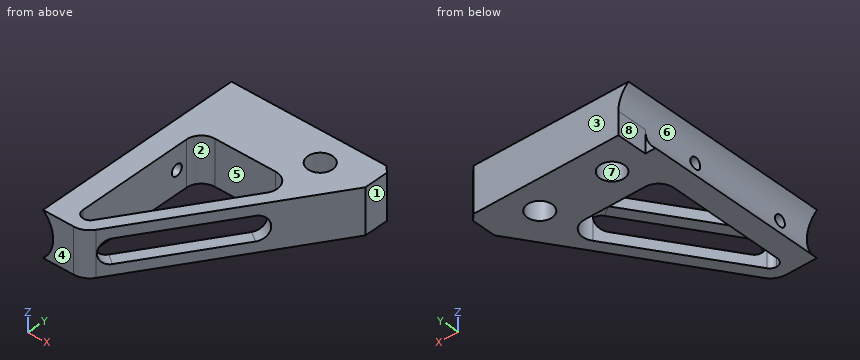
from build123d import *

# Parameters (mm, degrees)
P_IDAT_VYSUNUT_M1_DEPTH  = 15
SKICA3_R                 = 4.1
ODEBRAT_VYSUNUT_M1_DEPTH = 88.321245983
SKICA4_R                 = 4.05
ODEBRAT_VYSUNUT_M2_DEPTH = 10
ODEBRAT_VYSUNUT_M3_DEPTH = 88.321245983
P_IDAT_VYSUNUT_M2_DEPTH  = 70
SKICA7_W                 = 3.385621722
SKICA7_H                 = 7.5
ODEBRAT_VYSUNUT_M5_DEPTH = 10
SKICA9_W                 = 8
SKICA9_H                 = 44.544482181
ODEBRAT_VYSUNUT_M6_DEPTH = 88.290898193
ZAOBLIT2_R               = 4
SKICA10_R                = 1.85
ODEBRAT_VYSUNUT_M7_DEPTH = 86.094065598
ZAOBLIT7_R               = 6
ZKOSEN_1_SIZE            = 2


with BuildPart() as part:
    # Skica1 → Přidat vysunutím1 (new body)
    with BuildSketch(Plane.XY):
        Polygon((0, 0), (0, 70), (50, 70), (50, 60), (10, 0), align=None)
    extrude(amount=P_IDAT_VYSUNUT_M1_DEPTH)

    # Skica3 → Odebrat vysunutím1 (cut, through all)
    with BuildSketch(Plane.XY.offset(15)):
        with Locations((35, 60)):
            Circle(SKICA3_R)
    extrude(amount=-ODEBRAT_VYSUNUT_M1_DEPTH, mode=Mode.SUBTRACT)

    # Skica4 → Odebrat vysunutím2 (cut)
    with BuildSketch(Plane(origin=(0, 0, 0), x_dir=(-1, 0, 0), z_dir=(0, 0, -1))):
        with Locations((-11, 60)):
            Circle(SKICA4_R)
    extrude(amount=-ODEBRAT_VYSUNUT_M2_DEPTH, mode=Mode.SUBTRACT)

    # Skica5 → Odebrat vysunutím3 (cut, through all)
    with BuildSketch(Plane(origin=(0, 0, 0), x_dir=(-1, 0, 0), z_dir=(0, 0, -1))):
        with BuildLine():
            Line((-29.15001284, 49.95), (-9, 49.95))
            ThreePointArc((-9, 49.95), (-5.464466094, 48.485533906), (-4, 44.95))
            Line((-4, 44.95), (-4, 6.5))
            ThreePointArc((-4, 6.5), (-4.732233047, 4.732233047), (-6.5, 4))
            Line((-6.5, 4), (-6.52130557, 4))
            ThreePointArc((-6.52130557, 4), (-7.700950384, 4.295813503), (-8.601431306, 5.113249509))
            Line((-8.601431306, 5.113249509), (-33.310264312, 42.176499019))
            ThreePointArc((-33.310264312, 42.176499019), (-33.558385834, 47.309289628), (-29.15001284, 49.95))
        make_face()
    extrude(amount=-ODEBRAT_VYSUNUT_M3_DEPTH, mode=Mode.SUBTRACT)

    # Skica6 → Přidat vysunutím2 (add)
    with BuildSketch(Plane(origin=(0, 70, 0), x_dir=(1, 0, 0), z_dir=(0, 1, 0))):
        with BuildLine():
            Line((3.452933226, 0), (3.452933226, -15))
            Line((3.452933226, -15), (-3.385621722, -15))
            ThreePointArc((-3.385621722, -15), (0, -7.5), (-3.385621722, 0))
            Line((-3.385621722, 0), (3.452933226, 0))
        make_face()
    extrude(amount=-P_IDAT_VYSUNUT_M2_DEPTH)

    # Skica7 → Odebrat vysunutím5 (cut)
    with BuildSketch(Plane(origin=(0, 70, 0), x_dir=(1, 0, 0), z_dir=(0, 1, 0))):
        with Locations((-1.692810861, -3.75)):
            Rectangle(SKICA7_W, SKICA7_H)
    extrude(amount=-ODEBRAT_VYSUNUT_M5_DEPTH, mode=Mode.SUBTRACT)

    # Skica9 → Odebrat vysunutím6 (cut, through all)
    with BuildSketch(Plane(origin=(3.594875746, -2.39658383, 0), x_dir=(0, 0, 1), z_dir=(-0.8320502943378435, 0.5547001962252294, 0))):
        with Locations((7.5, 31.297937483)):
            Rectangle(SKICA9_W, SKICA9_H)
    extrude(amount=-ODEBRAT_VYSUNUT_M6_DEPTH, mode=Mode.SUBTRACT)

    # Zaoblit2
    zaoblit2_edges = [part.edges().sort_by_distance(p)[0] for p in [
        (10.265531894, 4.003849117, 11.5),
        (10.265531894, 4.003849117, 3.5),
        (34.974364901, 41.067098626, 3.5),
        (34.974364901, 41.067098626, 11.5),
    ]]
    fillet(zaoblit2_edges, radius=ZAOBLIT2_R - 0.0001)  # a hair under: the kernel refuses the full size

    # Skica10 → Odebrat vysunutím7 (cut, through all)
    with BuildSketch(Plane(origin=(4, 0, 0), x_dir=(0, 0, -1), z_dir=(1, 0, 0))):
        with Locations(Location((-7.5, 10, 0), (0, 0, 90))):
            Circle(SKICA10_R)
        with Locations(Location((-7.5, 41.45, 0), (0, 0, 90))):
            Circle(SKICA10_R)
    extrude(amount=-ODEBRAT_VYSUNUT_M7_DEPTH, mode=Mode.SUBTRACT)

    # Zaoblit7
    zaoblit7_edges = [part.edges().sort_by_distance(p)[0] for p in [
        (10, 0, 7.5),
    ]]
    fillet(zaoblit7_edges, radius=ZAOBLIT7_R)

    # Zkosení1
    zkosen_1_edges = [part.edges().sort_by_distance(p)[0] for p in [
        (50, 70, 7.5),
    ]]
    chamfer(zkosen_1_edges, length=ZKOSEN_1_SIZE)


solid = part.part
Geometry: final body of the model. Coordinates: model frame, mm. Face numbers are marked on the shaded views. A direction names the side the tool comes from. Give positions to 0.01 mm unless a question says otherwise; leave off trailing zeros. Write each loop counter-clockwise with the first axis right and the second up, starting at its lowest first coordinate (ties: lowest second). Pieces come first, ordered by that corner, then holes.
(1) Access query for the marked faces 5, 6, 7 and 8. Directions: +Z, -Z, +X, -X, +Y, -Y. A direction counts if a zero-diameter tool reaches every point of the face in a straight line with its end or side. Return the directions, or none.
(2) Cut plane A-A, the plane z = 6.5. Give the number of separate pieces and of enclosed holes in the cut face, then the cut area to 3 significant figures.
(3) Mould query, pull axis Y, two halves, no side actions, for the marked faces 1, 2, 3 and 4. Classes: released by +Y, released by -Y, zero draft, split by the parting line, or undercut.
(4) Cut plane C-C, the plane y = 26. Return loops of the section in (x, z).
(5) Ray query, line 1 (Y direction, x = 2.8, z = 7.5); line 2 (Z direction, x = 2, y = 10); line 3 (X direction, y = 66.5, z = 2.75). Return the intervals inside material, ascending.
(6) First-contact query: P1, Ø3, axis at x = 40, z = 6, coming from the -Y side; P2, Ø6, axis at y = 10, z = 7.5, coming from the +X side; P3, Ø4.5, axis at y = 24, z = 10.5, coming from the +X side. Flat tips, straight axial feed; report the tip coordinate or a pass-through.
(7) Cut plane D-D, the plane x = 45. Return loops of the section in (y, z), then the cut area to 4 significant figures.
(8) Cut plane B-B, the plane y = 10. Return loops of the section in (x, z).
Values follow:
1. face 5: +Z, -Z
1. face 6: -X, +Y, -Y
1. face 7: -Z
1. face 8: -Z, -X, +Y
2. separate pieces: 3
2. enclosed holes: 2
2. area: 1,140 mm2
3. face 1: zero draft
3. face 2: undercut
3. face 3: released by +Y
3. face 4: released by -Y
4. outline: (-3.39, 0) - (4, 0) - (4, 15) - (-3.39, 15) arc R10 cw to start; (22.53, 0) - (27.33, 0) - (27.33, 3.5) - (22.53, 3.5) - close; (22.53, 11.5) - (27.33, 11.5) - (27.33, 15) - (22.53, 15) - close
5. line 1: y = 0 to 8.15, 11.85 to 39.6, 43.3 to 70
5. line 2: z = 0 to 5.65, 9.35 to 15
5. line 3: x = 0 to 50
6. P1: stops at y = 42.75
6. P2: stops at x = 4
6. P3: stops at x = 27.34
7. outline: (52.5, 0) - (70, 0) - (70, 15) - (52.5, 15) - close
7. area: 262.5 mm2
8. outline: (-3.39, 0) - (4, 0) - (4, 5.65) - (-0.17, 5.65) arc R10 cw to start; (-3.39, 15) arc R10 cw to (-0.17, 9.35) - (4, 9.35) - (4, 15) - close; (11.86, 0) - (16.67, 0) - (16.67, 3.5) - (11.86, 3.5) - close; (11.86, 11.5) - (16.67, 11.5) - (16.67, 15) - (11.86, 15) - close
